Check sheet for the modelled part. Datum: model origin and axes. Units: mm. Round coordinates to 2 decimals unless told otherwise and drop trailing zeros. Write each loop counter-clockwise with the first axis right and the second up, starting at its lowest first coordinate (ties: lowest second). Pieces come first, ordered by that corner, then holes.
Item 1: Release check for a two-part mould opening along X. For faces 1 (the flat face through (2, 188, 0)), 2 (the cylindrical face through (-137.5, 207.4, 9.4)), 3 (the flat face through (-89.117, 139.242, 9.12)) record: pulls with the +X half, pulls with the -X half, needs draft (parallel to the pull), parting line crosses it, or undercut.
Item 2: Section check D-D, the plane x = 88.5. Record the cut outline in (y, z), plus the area to 3 significant figures.
Item 3: Depth check by flat-ended pin: pin 1 (6 mm diameter, centred on x = -65.5, z = 3, fed in from -Y); pin 2 (7 mm diameter, centred on x = 0, y = 90, fed in from +Z); pin 3 (9.5 mm diameter, centred on x = -136.14, y = 210.07, fed in from -Z); pin 4 (3 mm diameter, centred on y = 183, z = 7, fed in from +X). Enter the tip coordinate at first touch or a pass-through.
Item 4: Material ranges on line 1 along X through (y, z) = (216.5, 5); line 2 along Y through (x, z) = (134, 12.5); line 3 along X through (y, z) = (98, 16.5), recorded low to high.
Item 5: Section check A-A, the plane x = 0. Record the cut outline in (y, z), plus the area to 3 significant figures.
Item 6: Section check C-C, the plane y = 90. Record the cut outline in (x, z).
Item 7: Section check B-B, the plane z = 10.5. Record the cut outline in (x, y).
from build123d import *

# Parameters (mm, degrees)
SKETCH_R          = 4.25
PAD_DEPTH         = 18.5
SKETCH001_R       = 3
POCKET_DEPTH      = 799.519554
POCKET_DEPTH_BACK = 818.019554


with BuildPart() as part:
    # Sketch → Pad (new body)
    with BuildSketch(Plane.XY):
        with BuildLine():
            Line((-170.743902, 224.737113), (-117.916352, 255.237113))
            ThreePointArc((-107.916352, 257.916605), (-113.092733, 257.235122), (-117.916352, 255.237113))
            Line((-107.916352, 257.916605), (107.916352, 257.916605))
            ThreePointArc((117.916352, 255.237113), (113.092733, 257.235122), (107.916352, 257.916605))
            Line((117.916352, 255.237113), (170.743902, 224.737113))
            ThreePointArc((172.135351, 201.406349), (177.719069, 213.446238), (170.743902, 224.737113))
            Line((172.135351, 201.406349), (8.391449, 78.793592))
            ThreePointArc((-8.391449, 78.793592), (0, 76), (8.391449, 78.793592))
            Line((-8.391449, 78.793592), (-172.135351, 201.406349))
            ThreePointArc((-170.743902, 224.737113), (-177.719069, 213.446238), (-172.135351, 201.406349))
        make_face()
        with Locations((163.743902, 212.612757)):
            Circle(SKETCH_R, mode=Mode.SUBTRACT)
        with Locations((-163.743902, 212.612757)):
            Circle(SKETCH_R, mode=Mode.SUBTRACT)
        with Locations((0, 90)):
            Circle(SKETCH_R, mode=Mode.SUBTRACT)
    extrude(amount=PAD_DEPTH)

    # Sketch001 → Pocket (cut, two sides)
    with BuildSketch(Plane.XY) as pocket_sk:
        with Locations((113.858583, 222.938851)):
            Circle(SKETCH001_R)
        with Locations((136.141417, 210.073851)):
            Circle(SKETCH001_R)
    pocket = extrude(amount=-POCKET_DEPTH, mode=Mode.SUBTRACT) + extrude(pocket_sk.sketch, amount=POCKET_DEPTH_BACK, mode=Mode.SUBTRACT)

    # Mirrored: Pocket across Sketch001 V_Axis
    add(pocket.mirror(Plane(origin=(0, 0, 0), x_dir=(0, 0, 1), z_dir=(1, 0, 0))), mode=Mode.SUBTRACT)


solid = part.part
Values found:
1. face 1: needs draft
1. face 2: undercut
1. face 3: pulls with the -X half
2. outline: (138.78, 0) - (257.92, 0) - (257.92, 18.5) - (138.78, 18.5) - close
2. area: 2,200 mm2
3. pin 1: stops at y = 119.31
3. pin 2: passes through
3. pin 3: stops at z = 0
3. pin 4: stops at x = 149.56
4. line 1: x = -177.19 to -165.46, -162.03 to 162.03, 165.46 to 177.19
4. line 2: y = 172.85 to 207.97, 212.17 to 245.95
4. line 3: x = -34.04 to 34.04
5. outline: (76, 0) - (85.75, 0) - (85.75, 18.5) - (76, 18.5) - close; (94.25, 0) - (257.92, 0) - (257.92, 18.5) - (94.25, 18.5) - close
5. area: 3,210 mm2
6. outline: (-23.36, 0) - (-4.25, 0) - (-4.25, 18.5) - (-23.36, 18.5) - close; (4.25, 0) - (23.36, 0) - (23.36, 18.5) - (4.25, 18.5) - close
7. outline: (-172.14, 201.41) - (-8.39, 78.79) arc R14 ccw to (8.39, 78.79) - (172.14, 201.41) arc R14 ccw to (170.74, 224.74) - (117.92, 255.24) arc R20 ccw to (107.92, 257.92) - (-107.92, 257.92) arc R20 ccw to (-117.92, 255.24) - (-170.74, 224.74) arc R14 ccw to start; hole circle Ø8.5 at (-163.74, 212.61); hole circle Ø6 at (-136.14, 210.07); hole circle Ø6 at (-113.86, 222.94); hole circle Ø8.5 at (0, 90); hole circle Ø6 at (113.86, 222.94); hole circle Ø6 at (136.14, 210.07); hole circle Ø8.5 at (163.74, 212.61)
